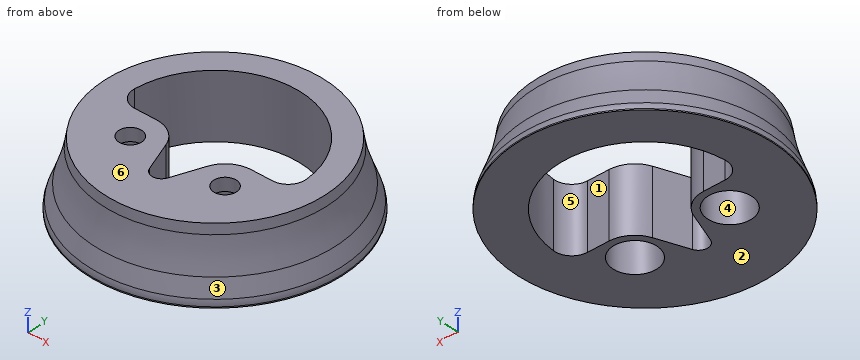
```python
from build123d import *

# Parameters (mm, degrees)
F2_R     = 2.625
F3_DEPTH = 15.001
F4_R     = 5.075
F5_DEPTH = 12


with BuildPart() as f1:
    # F0 (on Front) → F1 (revolve)
    with BuildSketch(Plane.XZ):
        with BuildLine():
            Line((-29.5, 0.274662), (-29.5, 0))
            Line((-29.5, 0), (0, 0))
            Line((0, 0), (0, 15))
            Line((0, 15), (-25.5, 15))
            Line((-25.5, 15), (-25.861378, 12.831729))
            ThreePointArc((-25.861378, 12.831729), (-26.681762, 9.048734), (-27.863968, 5.362751))
            Line((-27.863968, 5.362751), (-29.245317, 1.679155))
            ThreePointArc((-29.245317, 1.679155), (-29.435814, 0.988361), (-29.5, 0.274662))
        make_face()
    revolve(axis=Axis((0, 0, 21.150352), (0, 0, 1)))

    # F2 (on face) → F3 (cut, through all)
    with BuildSketch(Plane.XY.offset(15)):
        with BuildLine():
            ThreePointArc((15.9604, -2.875), (18.886575, -1.602178), (19.9505, 1.40625))
            ThreePointArc((19.9505, 1.40625), (0, 20), (-19.9505, 1.40625))
            ThreePointArc((-19.9505, 1.40625), (-18.886575, -1.602178), (-15.9604, -2.875))
            Line((-15.9604, -2.875), (-11, -2.875))
            ThreePointArc((-11, -2.875), (-7.224013, -4.056421), (-4.794753, -7.179325))
            Line((-4.794753, -7.179325), (-2.107442, -14.364916))
            ThreePointArc((-2.107442, -14.364916), (0, -15.826762), (2.107442, -14.364916))
            Line((2.107442, -14.364916), (4.794753, -7.179325))
            ThreePointArc((4.794753, -7.179325), (7.224013, -4.056421), (11, -2.875))
            Line((11, -2.875), (15.9604, -2.875))
        make_face()
        with Locations((-11, -9.5)):
            Circle(F2_R)
        with Locations((11, -9.5)):
            Circle(F2_R)
    extrude(amount=-F3_DEPTH, mode=Mode.SUBTRACT)

    # F4 (on face) → F5 (cut)
    with BuildSketch(Plane(origin=(0, 0, 0), x_dir=(1, 0, 0), z_dir=(0, 0, -1))):
        with Locations((11, 9.5)):
            Circle(F4_R)
        with Locations((-11, 9.5)):
            Circle(F4_R)
    extrude(amount=-F5_DEPTH, mode=Mode.SUBTRACT)


solid = f1.part
```
Check sheet for the modelled part. Datum: model origin and axes. Units: mm. Face numbers are marked on the shaded views. A direction names the side the tool comes from. Round coordinates to 2 decimals unless told otherwise and drop trailing zeros. Order: outer loops, then holes, each group sorted by start corner. A loop starts at its lowest first (then second) coordinate and runs counter-clockwise, first axis right, second up. Notation, with made-up numbers: (56.5, 86.25) -> (111.5, 86.25) arc R9 cw to (111.5, 101.25) -> close; hole circle Ø11 at (35, -10). An arc over 180 degrees is marked (long way). One line per item, written item: value. Start each with the question number.
Q1. Cross-section at A-A (x = 0). Record the boundary of the cut face in (y, z), and give its area (3 significant figures).
Q2. Cross-section at C-C (z = 7.75). Give the number of separate pieces and of enclosed holes in the cut face, and give its area (3 significant figures).
Q3. Mould release check, pull along Y, two halves, no side actions. Record for the marked faces 1, 2 and 3: pulls with the +Y half, pulls with the -Y half, needs draft (parallel to the pull), parting line crosses it, or undercut.
Q4. Thickness scan on line 1 (Y direction, x = -11, z = 14) (3 decimals); line 2 (X direction, y = -9.5, z = 4) (3 decimals); line 3 (Y direction, x = -11, z = 13.6) (3 decimals). Record the ranges inside material, lowest first.
Q5. Cross-section at B-B (y = 0). Record the boundary of the cut face in (x, z), and give its area (3 significant figures).
Q6. Gauge pin test, flat ends, axial feed: pin 1 Ø1.5 at (x, z) = (-11.5, 11.5) entering from -Y; pin 2 Ø1.5 at (y, z) = (-9, 10) entering from +X; pin 3 Ø1.5 at (x, z) = (14.5, 5.5) entering from +Y. Record the tip position at first contact, or that the pin passes through.
Q7. Set-up check for the marked faces 4, 5 and 6: record each of +Z, -Z, +X, -X, +Y, -Y from which the full face is reachable in a straight line by a thin tool's end or side.
Completed:
1. outline: (-29.5, 0) -> (-15.83, 0) -> (-15.83, 15) -> (-25.5, 15) -> (-25.86, 12.83) arc R40 cw to (-27.86, 5.36) -> (-29.25, 1.68) arc R4 ccw to (-29.5, 0.27) -> close; (20, 0) -> (29.5, 0) -> (29.5, 0.27) arc R4 ccw to (29.25, 1.68) -> (27.86, 5.36) arc R40 cw to (25.86, 12.83) -> (25.5, 15) -> (20, 15) -> close
1. area: 283 mm²
2. separate pieces: 1
2. enclosed holes: 3
2. area: 1,290 mm²
3. face 1: undercut
3. face 2: needs draft
3. face 3: parting line crosses it
4. line 1: y = -23.19 to -12.125, -6.875 to -2.875, 16.703 to 23.19
4. line 2: x = -26.737 to -16.075, -5.925 to -3.927, 3.927 to 5.925, 16.075 to 26.737
4. line 3: y = -23.264 to -12.125, -6.875 to -2.875, 16.703 to 23.264
5. outline: (-29.5, 0) -> (-19.8, 0) -> (-19.8, 15) -> (-25.5, 15) -> (-25.86, 12.83) arc R40 cw to (-27.86, 5.36) -> (-29.25, 1.68) arc R4 ccw to (-29.5, 0.27) -> close; (19.8, 0) -> (29.5, 0) -> (29.5, 0.27) arc R4 ccw to (29.25, 1.68) -> (27.86, 5.36) arc R40 cw to (25.86, 12.83) -> (25.5, 15) -> (19.8, 15) -> close
5. area: 226 mm²
6. pin 1: stops at y = -23.83
6. pin 2: stops at x = 25.19
6. pin 3: stops at y = 24.28
7. face 4: -Z
7. face 5: +Z, -Z
7. face 6: +Z, +X, -X, +Y, -Y
